Autodesk Inventor part; units mm, degrees
ref_plane "YZ Plane" through (0, 0, 0) normal (1, 0, 0) x (0, 1, 0)
ref_plane "XZ Plane" through (0, 0, 0) normal (0, 1, 0) x (-1, 0, 0)
ref_plane "XY Plane" through (0, 0, 0) normal (0, 0, 1) x (1, 0, 0)
sketch "Vertical" plane through (0, 0, 0) normal (0, 0, 1) x (1, 0, 0)
  line L0 (10, -3) -> (-10, -3)
  line L1 (-10, -3) -> (-10, 3)
  line L2 (-10, 3) -> (10, 3)
  line L3 (10, 3) -> (10, -3)
  line L4 (10, -3) -> (-10, 3) construction
  line L5 (-10, -3) -> (10, 3) construction
  line L6 (-10, 3) -> (-6.1, 17)
  arc A0 (6.1, 17) -> (-6.1, 17) centre (0, 17) ccw
  line L7 (6.1, 17) -> (10, 3)
  line L8 (0, -8.22) -> (0, 28.32)
  circle A1 centre (0, 17) radius 2.1
  line L9 (-6.1, 17) -> (6.1, 17)
  circle A2 centre (0, 17) radius 4.1
  line L10 (-4.1569, 17) -> (-2.0785, 20.6)
  line L11 (-2.0785, 20.6) -> (2.0785, 20.6)
  line L12 (2.0785, 20.6) -> (4.1569, 17)
  line L13 (4.1569, 17) -> (2.0785, 13.4)
  line L14 (2.0785, 13.4) -> (-2.0785, 13.4)
  line L15 (-2.0785, 13.4) -> (-4.1569, 17)
  point P0 (0, 0)
  point P1 (0, 0)
  point P2 (-1.9621, 20.6)
  point P3 (-2.1366, 20.4993)
  point P4 (4.0988, 17.1007)
  point P5 (4.0988, 16.8993)
  point P6 (2.1366, 20.4993)
  point P7 (1.9621, 20.6)
  point P8 (1.9621, 13.4)
  point P9 (2.1366, 13.5007)
  point P10 (-2.1366, 13.5007)
  point P11 (-1.9621, 13.4)
  point P12 (-4.0988, 16.8993)
  point P13 (-4.0988, 17.1007)
  dimension "d6" = 6
  dimension "d7" = 20
  dimension "d8" = 14
  dimension "d9" = 4.2
  dimension "d10" = 4
  dimension "d11" = 8.2
  dimension "d12" = 20
  dimension "d34" = 7.2
extrude "Extrusion1" add sketch "Vertical" along normal mid plane 16 contours L2 L8 A2 L14 L13 L9 L7 | L2 L6 L9 L15 A2 L14 L8 | L9 L12 A2 L11 L8 A0 | A2 L14 L8 | L8 L14 A2 | L8 A2 L11 L10 L9 A0 | L13 A2 L9 | L9 A2 L12 | L14 A2 L15 L9 A1 L8 | L8 A1 L9 A2 L13 L14 | L14 L15 A2 | A2 L13 L14 | A2 L11 L8 | L8 L11 A2 | L9 A1 L8 L11 A2 L12 | L12 A2 | A2 L13 | L10 A2 L9 | L9 A2 L15 | A2 L15 | L8 A1 L9 A2 L10 L11 | L11 L12 A2 | A2 L10 L11 | A2 L10
extrude "Extrusion6" cut sketch "Vertical" against normal through all contours A2 L14 L8 | L8 L14 A2 | L14 A2 L15 L9 A1 L8 | L8 A1 L9 A2 L13 L14 | A2 L11 L8 | L8 L11 A2 | L9 A1 L8 L11 A2 L12 | L12 A2 | A2 L13 | A1 L9 L8 | L8 L9 A1 | A2 L15 | L8 A1 L9 A2 L10 L11 | L9 L8 A1 | A2 L10 | L9 A1 L8
extrude "Extrusion8" cut sketch "Vertical" along normal through all contours L13 A2 L9 | L9 A2 L12 | L14 A2 L15 L9 A1 L8 | L8 A1 L9 A2 L13 L14 | L14 L15 A2 | A2 L13 L14 | L9 A1 L8 L11 A2 L12 | L10 A2 L9 | L9 A2 L15 | A1 L9 L8 | L8 L9 A1 | L8 A1 L9 A2 L10 L11 | L11 L12 A2 | A2 L10 L11 | L9 L8 A1 | L9 A1 L8
extrude "Extrusion7" add sketch "Vertical" along normal mid plane 12 contours A2 L14 L8 | L8 L14 A2 | L13 A2 L9 | L9 A2 L12 | L14 A2 L15 L9 A1 L8 | L8 A1 L9 A2 L13 L14 | L14 L15 A2 | A2 L13 L14 | A2 L11 L8 | L8 L11 A2 | L9 A1 L8 L11 A2 L12 | L12 A2 | A2 L13 | L10 A2 L9 | L9 A2 L15 | A2 L15 | L8 A1 L9 A2 L10 L11 | L11 L12 A2 | A2 L10 L11 | A2 L10
extrude "Extrusion2" cut sketch "Vertical" along normal mid plane 6 contours L2 L8 A2 L14 L13 L9 L7 | L2 L6 L9 L15 A2 L14 L8 | L9 L12 A2 L11 L8 A0 | A2 L14 L8 | L8 L14 A2 | L8 A2 L11 L10 L9 A0 | L13 A2 L9 | L9 A2 L12 | L14 A2 L15 L9 A1 L8 | L8 A1 L9 A2 L13 L14 | L14 L15 A2 | A2 L13 L14 | A2 L11 L8 | L8 L11 A2 | L9 A1 L8 L11 A2 L12 | L12 A2 | A2 L13 | L10 A2 L9 | L9 A2 L15 | A1 L9 L8 | L8 L9 A1 | A2 L15 | L8 A1 L9 A2 L10 L11 | L11 L12 A2 | A2 L10 L11 | L9 L8 A1 | A2 L10 | L9 A1 L8
sketch "Horizontale" plane through (-10, 3, 8) normal (0, -1, 0) x (1, 0, 0)
  line L0 (0, -5) -> (20, -5)
  line L1 (20, -5) -> (20, 0)
  line L2 (0, 0) -> (20, 0)
  line L3 (0, -5) -> (0, 0)
  line L4 (20, -11) -> (0, -11)
  line L5 (0, -16) -> (0, -11)
  line L6 (20, -16) -> (0, -16)
  line L7 (20, -16) -> (20, -11)
  line L8 (20, -8) -> (0, -8)
  line L9 (0, -22.5) -> (20, -22.5)
  line L10 (20, -22.5) -> (20, 6.5)
  line L11 (20, 6.5) -> (0, 6.5)
  line L12 (0, 6.5) -> (0, -22.5)
  line L13 (0, -22.5) -> (20, 6.5) construction
  line L14 (20, -22.5) -> (0, 6.5) construction
  line L15 (4, -18.75) -> (16, -18.75) construction
  line L16 (16, -18.75) -> (16, 2.75) construction
  line L17 (16, 2.75) -> (4, 2.75) construction
  line L18 (4, 2.75) -> (4, -18.75) construction
  line L19 (4, -18.75) -> (16, 2.75) construction
  line L20 (16, -18.75) -> (4, 2.75) construction
  circle A0 centre (16, 2.75) radius 1.5
  circle A1 centre (4, 2.75) radius 1.5
  circle A2 centre (16, -18.75) radius 1.5
  circle A3 centre (4, -18.75) radius 1.5
  line L21 (14.4123, 0) -> (12.8246, 2.75)
  line L22 (12.8246, 2.75) -> (14.4123, 5.5)
  line L23 (14.4123, 5.5) -> (17.5877, 5.5)
  line L24 (17.5877, 5.5) -> (19.1754, 2.75)
  line L25 (19.1754, 2.75) -> (17.5877, 0)
  line L26 (17.5877, 0) -> (14.4123, 0)
  line L27 (2.4123, 0) -> (0.8246, 2.75)
  line L28 (0.8246, 2.75) -> (2.4123, 5.5)
  line L29 (2.4123, 5.5) -> (5.5877, 5.5)
  line L30 (5.5877, 5.5) -> (7.1754, 2.75)
  line L31 (7.1754, 2.75) -> (5.5877, 0)
  line L32 (5.5877, 0) -> (2.4123, 0)
  line L33 (5.5877, -16) -> (7.1754, -18.75)
  line L34 (7.1754, -18.75) -> (5.5877, -21.5)
  line L35 (5.5877, -21.5) -> (2.4123, -21.5)
  line L36 (2.4123, -21.5) -> (0.8246, -18.75)
  line L37 (0.8246, -18.75) -> (2.4123, -16)
  line L38 (2.4123, -16) -> (5.5877, -16)
  line L39 (17.5877, -16) -> (19.1754, -18.75)
  line L40 (19.1754, -18.75) -> (17.5877, -21.5)
  line L41 (17.5877, -21.5) -> (14.4123, -21.5)
  line L42 (14.4123, -21.5) -> (12.8246, -18.75)
  line L43 (12.8246, -18.75) -> (14.4123, -16)
  line L44 (14.4123, -16) -> (17.5877, -16)
  point P0 (10, -8)
  point P1 (16, 0)
  point P2 (4, 0)
  point P3 (4, -16)
  point P4 (16, -16)
  point P5 (2.4123, 0)
  point P6 (5.5877, 0)
  point P7 (2.4123, -16)
  point P8 (14.4123, 0)
  point P9 (17.5877, 0)
  dimension "d17" = 5.5
  dimension "d18" = 3
  dimension "d19" = 1
  dimension "d20" = 12
  dimension "d21" = 21.5
  dimension "d28" = 6
extrude "Extrusion3" add sketch "Horizontale" along normal blind 6 contours L3 L2 L1 L0 | L0 L10 L8 L12 | L12 L11 L10 L2 L25 L24 L23 L22 L21 L31 L30 L29 L28 L27 | L8 L10 L4 L12 | L27 L28 L29 L30 L31 L2 | L4 L7 L6 L5 | L2 L21 L22 L23 L24 L25 | L6 L37 L36 L35 L34 L33 L43 L42 L41 L40 L39 L10 L9 L12 | L6 L33 L34 L35 L36 L37 | L39 L40 L41 L42 L43 L6 | A0 | A1 | A2 | A3
extrude "Extrusion4" cut sketch "Horizontale" along normal through all contours A0 | A1 | A2 | A3
extrude "Extrusion5" cut sketch "Horizontale" along normal blind 3.5 contours L27 L28 L29 L30 L31 L2 | L2 L21 L22 L23 L24 L25 | L6 L33 L34 L35 L36 L37 | L39 L40 L41 L42 L43 L6
fillet "Congé1" radius 2 4 edges at (10, 0, 14.5) (-10, 0, 14.5) (10, 0, -14.5) (-10, 0, -14.5)
properties part number "Support rotation"
Design review of the part built by this model. Coordinates are the model's own, in mm. A direction names the side the tool comes from. Round coordinates to 2 decimals unless told otherwise and drop trailing zeros. Write each loop counter-clockwise with the first axis right and the second up, starting at its lowest first coordinate (ties: lowest second). Pieces come first, ordered by that corner, then holes.
Item 1: Draft analysis for pull direction Z (two halves, no side actions). For faces 1 (the flat face through (8.37, 1.274, 12.144)), 2 (the flat face through (2, 15, -6)), 3 (the cylindrical face through (9.43, -0.04, 13.9)), state which applies: released by +Z, released by -Z, zero draft, split by the parting line, or undercut.
Item 2: Consider section A-A on x = 0. Give the boundary of the cut face in (y, z).
Item 3: Wall thickness on L1, parallel to Z at x = 6, y = -1.9; L2, parallel to X at y = -1.3, z = -10.75; L3, parallel to Z at x = -5.5, y = 1.25: over which ranges is each line inside the solid? List them lowest first.
Item 4: Consider section C-C on z = -10. Give the boundary of the cut face in (x, y), and give its area (3 significant figures).
Item 5: Consider section B-B on y = 14.25. Give the boundary of the cut face in (x, z).
Item 6: Consider section D-D on y = 10.5. Give the boundary of the cut face in (x, z).
Item 7: For faces 4 (the flat face through (0, 3, -11)), 5 (the flat face through (8.37, 1.274, -9.356)), 6 (the flat face through (0, 3, 11)), list the 3-axis set-ups (+Z, -Z, +X, -X, +Y, -Y) from which the entire face can be reached by the end or side of a thin tool; tool diameter is ignored.
Item 8: For pin 1 Ø1 at (x, z) = (3, 4) entering from +Y; pin 2 Ø10.5 at (x, y) = (0, 17) entering from +Z; pin 3 Ø6.5 at (x, y) = (-0.5, 18.5) entering from -Z, all flat-tipped, find the tip position at first contact; note any pin that passes through.
Check values:
1. face 1: undercut
1. face 2: released by -Z
1. face 3: released by +Z
2. outline: (-3, -14.5) - (3, -14.5) - (3, -8) - (12.9, -8) - (12.9, -6) - (14.9, -6) - (14.9, -3) - (3, -3) - (3, 3) - (14.9, 3) - (14.9, 6) - (13.4, 6) - (13.4, 8) - (3, 8) - (3, 14.5) - (-3, 14.5) - close; (19.1, -6) - (21.1, -6) - (21.1, -8) - (23.1, -8) - (23.1, -3) - (19.1, -3) - close; (19.1, 3) - (23.1, 3) - (23.1, 8) - (20.6, 8) - (20.6, 6) - (19.1, 6) - close
3. L1: z = -14.5 to -12.25, -9.25 to 9.25, 12.25 to 14.5
3. L2: x = -10 to -7.5, -4.5 to 4.5, 7.5 to 10
3. L3: z = -14.5 to -13.5, -8 to 8, 13.5 to 14.5
4. outline: (-10, -3) - (-7.3, -3) - (-7.3, -0.5) - (-8.74, -0.5) - (-8.74, 3) - (-10, 3) - close; (-4.7, -3) - (4.7, -3) - (4.7, -0.5) - (3.26, -0.5) - (3.26, 3) - (-3.26, 3) - (-3.26, -0.5) - (-4.7, -0.5) - close; (7.3, -3) - (10, -3) - (10, 3) - (8.74, 3) - (8.74, -0.5) - (7.3, -0.5) - close
4. area: 68.6 mm2
5. outline: (-6.87, -8) - (-3.04, -8) - (-3.04, -6) - (3.04, -6) - (3.04, -8) - (6.87, -8) - (6.87, -3) - (-6.87, -3) - close; (-6.87, 3) - (6.87, 3) - (6.87, 8) - (2.57, 8) - (2.57, 6) - (-2.57, 6) - (-2.57, 8) - (-6.87, 8) - close
6. outline: (-7.91, -8) - (7.91, -8) - (7.91, -3) - (-7.91, -3) - close; (-7.91, 3) - (7.91, 3) - (7.91, 8) - (-7.91, 8) - close
7. face 4: -Z, +X, -X, +Y
7. face 5: +Y
7. face 6: +Z, +X, -X, +Y
8. pin 1: stops at y = 22.56
8. pin 2: stops at z = 8
8. pin 3: stops at z = -8
